Geometry check sheet. Reference: the model listing, model coordinates, mm. A direction names the side the tool comes from. Coordinates: 2 decimals unless noted, no trailing zeros. Loops run counter-clockwise (first coordinate to the right, second up) from the corner with the lowest first, then second, coordinate; pieces in that order, holes last. Notation, with made-up numbers: (4.25, 82.25) - (21.25, 82.25) arc R23 cw to (21.25, 94.25) - close; hole circle Ø7 at (2, 14.5). An arc over 180 degrees is marked (long way). Write each question's results on one line, items separated by ' | '. Start each with the question number.
(1) Go/stop test with flat-tipped pins: pin 1 Ø6.5 at (x, y) = (516, 10) entering from +Z; pin 2 Ø2 at (x, y) = (77, 1.5) entering from -Z; pin 3 Ø4.5 at (x, y) = (501, 8) entering from +Z. Record where each tip stops, or that it passes through.
(2) Sectioned sample at B-B (y = 12). Enter the section's corners in (x, z), plus the area to 3 significant figures.
(3) Sectioned sample at A-A (z = 24.5). Enter the section's corners in (x, y), plus the area to 3 significant figures.
(4) Access from +Z, -Z, +X, -X, +Y, -Y to the whole of each face (thin tool, end or side, straight path). Record for faces 4 (the face through (273, 15, 33)), 5 (the face through (-4, 8, 20)), 6 (the face through (20, 7, 25)), 7 (the face through (480, 7, 15)), 8 (the face through (514, 8, 20)).
(5) Sectioned sample at C-C (x = 153.5). Enter the section's corners in (y, z).
(6) Mould release check, pull along X, two halves, no side actions. Record for faces 1 (the face through (500, 8, 10)), 2 (the face through (11, 8, 0)), 3 (the face through (518, 7, 10)): pulls with the +X half, pulls with the -X half, needs draft (parallel to the pull), parting line crosses it, or undercut.
(7) Material ranges on probe 1 along X at (y, z) = (8.25, 12.5); probe 2 along X at (y, z) = (14, 4); probe 3 along X at (y, z) = (7, 28), recorded low to high.
from build123d import *

# Parameters (mm, degrees)
SKETCH_1_W           = 510
SKETCH_1_H           = 15
EXTRUDE_1_DEPTH      = 10
EXTRUDE_2_DEPTH      = 10
EXTRUDE_2_DEPTH_BACK = 10
SKETCH_2_W           = 8
SKETCH_2_H           = 15
EXTRUDE_3_DEPTH      = 15
SKETCH_4_W           = 450
SKETCH_4_H           = 10
CUT_EXTRUDE_1_DEPTH  = 520.758597812


with BuildPart() as part:
    # 草图1 → 凸台-拉伸1 (new body)
    with BuildSketch(Plane.XY):
        with Locations((255, 7.5)):
            Rectangle(SKETCH_1_W, SKETCH_1_H)
    extrude(amount=EXTRUDE_1_DEPTH)

    # 草图2 → 凸台-拉伸2 (add, two sides: drawn at the far end of the back side and taken through both)
    with BuildSketch(Plane.XY.offset(10).offset(-EXTRUDE_2_DEPTH_BACK)):
        with Locations((514, 7.5)):
            Rectangle(SKETCH_2_W, SKETCH_2_H)
        with Locations((-4, 7.5)):
            Rectangle(SKETCH_2_W, SKETCH_2_H)
    extrude(amount=EXTRUDE_2_DEPTH + EXTRUDE_2_DEPTH_BACK)

    # 草图3 → 凸台-拉伸3 (add)
    with BuildSketch(Plane.XZ):
        Polygon((20, 40), (20, 10), (30, 10), (30, 30), (480, 30), (480, 10), (490, 10), (490, 40), align=None)
    extrude(amount=-EXTRUDE_3_DEPTH)

    # 草图4 → 切除-拉伸1 (cut, through all)
    with BuildSketch(Plane.XZ):
        with Locations((255, 5)):
            Rectangle(SKETCH_4_W, SKETCH_4_H)
    extrude(amount=-CUT_EXTRUDE_1_DEPTH, mode=Mode.SUBTRACT)


solid = part.part
Outcome:
1) pin 1: stops at z = 20 | pin 2: stops at z = 30 | pin 3: stops at z = 10
2) outline: (-8, 0) - (30, 0) - (30, 30) - (480, 30) - (480, 0) - (518, 0) - (518, 20) - (510, 20) - (510, 10) - (490, 10) - (490, 40) - (20, 40) - (20, 10) - (0, 10) - (0, 20) - (-8, 20) - close | area: 6,020 mm2
3) outline: (20, 0) - (30, 0) - (30, 15) - (20, 15) - close; (480, 0) - (490, 0) - (490, 15) - (480, 15) - close | area: 300 mm2
4) face 4: +Z, -Z, +X, -X, +Y | face 5: +Z, -X, +Y, -Y | face 6: +Z, +Y, -Y | face 7: -Z, +Y, -Y | face 8: +Z, +X, +Y, -Y
5) outline: (0, 30) - (15, 30) - (15, 40) - (0, 40) - close
6) face 1: undercut | face 2: needs draft | face 3: pulls with the +X half
7) probe 1: x = -8 to 0, 20 to 30, 480 to 490, 510 to 518 | probe 2: x = -8 to 30, 480 to 518 | probe 3: x = 20 to 30, 480 to 490
